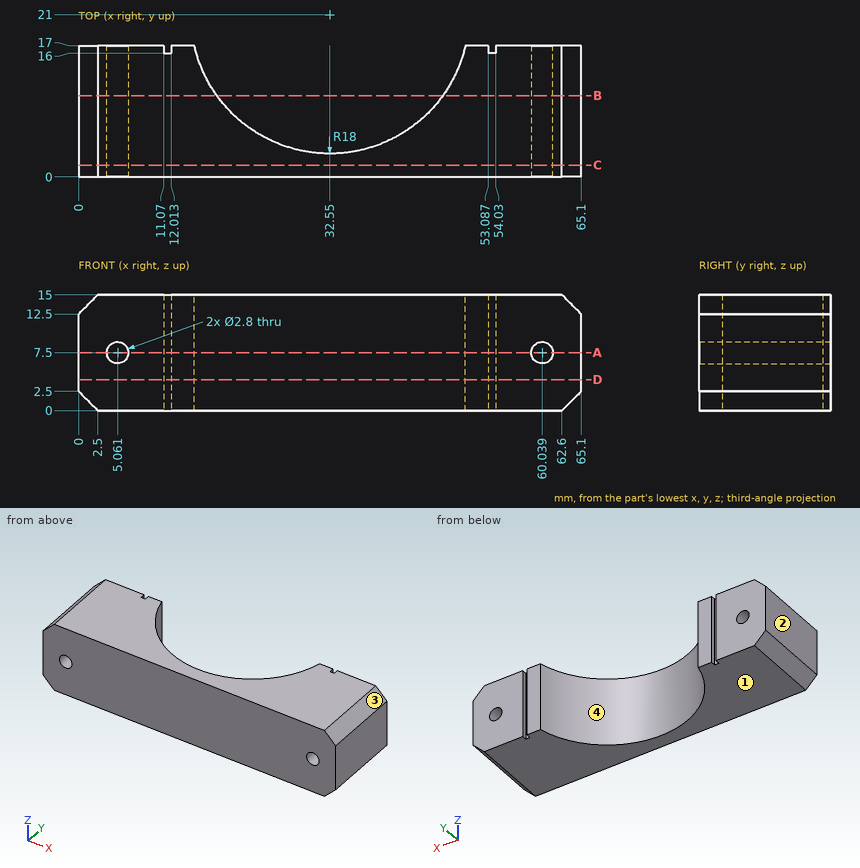
Design review of the part shown in the three views and the two pictorial views. Dimensions are in mm from the part's minimum x, y and z. Coordinates: 2 decimals unless noted, no trailing zeros. Loops run counter-clockwise (first coordinate to the right, second up) from the corner with the lowest first, then second, coordinate; pieces in that order, holes last.
Q1. We need section C-C on y = 1.5. State the section outline as (x, z) points.
Reported:
outline: (0, 2.5) - (2.5, 0) - (62.6, 0) - (65.1, 2.5) - (65.1, 12.5) - (62.6, 15) - (2.5, 15) - (0, 12.5) - close; hole circle Ø2.8 at (5.06, 7.5); hole circle Ø2.8 at (60.04, 7.5)
Q2. We need section B-B on y = 10.5. State the section outline as (x, z) points.
Reported:
outline: (0, 2.5) - (2.5, 0) - (17.93, 0) - (17.93, 15) - (2.5, 15) - (0, 12.5) - close; (47.17, 0) - (62.6, 0) - (65.1, 2.5) - (65.1, 12.5) - (62.6, 15) - (47.17, 15) - close; hole circle Ø2.8 at (5.06, 7.5); hole circle Ø2.8 at (60.04, 7.5)
Q3. We need section A-A on z = 7.5. State the section outline as (x, y) points.
Reported:
outline: (0, 0) - (3.66, 0) - (3.66, 17) - (0, 17) - close; (6.46, 0) - (58.64, 0) - (58.64, 17) - (54.03, 17) - (54.03, 16) - (53.09, 16) - (53.09, 17) - (50.1, 17) arc R18 cw to (15, 17) - (12.01, 17) - (12.01, 16) - (11.07, 16) - (11.07, 17) - (6.46, 17) - close; (61.44, 0) - (65.1, 0) - (65.1, 17) - (61.44, 17) - close
Q4. To check wall thickness, follow line 1 (X direction, y = 14.75, z = 8) (1 decimal); line 2 (X direction, y = 8.75, z = 12); line 3 (X direction, y = 9.25, z = 4.25) (1 decimal). State the ranges of each line that lie inside material, in increasing order.
Reported:
line 1: x = 0 to 3.8, 6.4 to 15.7, 49.4 to 58.7, 61.3 to 65.1
line 2: x = 0 to 19.36, 45.74 to 65.1
line 3: x = 0 to 18.9, 46.2 to 65.1
Q5. The part is to be moulded in two halves that separate along X. For the marked faces 1, 2, 3 and 4, say which applies: +X half, -X half, draft (parallel to the pull), parting line (faces both ways), or undercut.
Reported:
face 1: draft
face 2: -X half
face 3: +X half
face 4: undercut
Q6. For pin 1 (0.5 mm diameter, centred on x = 11.5, z = 4.5, fed in from +Y), flat-tipped, find the tip position at first contact; note if it passes through.
Reported:
pin 1: stops at y = 16
Q7. We need section D-D on z = 4. State the section outline as (x, y) points.
Reported:
outline: (0, 0) - (65.1, 0) - (65.1, 17) - (54.03, 17) - (54.03, 16) - (53.09, 16) - (53.09, 17) - (50.1, 17) arc R18 cw to (15, 17) - (12.01, 17) - (12.01, 16) - (11.07, 16) - (11.07, 17) - (0, 17) - close
